Can you work these out from the model? Positions are in its coordinate system, mm. Face numbers are marked on the shaded views. A direction names the side the tool comes from. Give positions to 0.01 mm unless a question says otherwise; leave off trailing zeros. Order: outer loops, then holes, each group sorted by start corner. A loop starts at its lowest first (then second) coordinate and runs counter-clockwise, first axis right, second up. Notation, with made-up numbers: (-12, -1.5) - (-4, -1.5) arc R17 cw to (-4, 31.5) - close; hole circle Ø7 at (-26.5, -29). An arc over 180 degrees is marked (long way). Return JSON: item names as keys, results as strings.
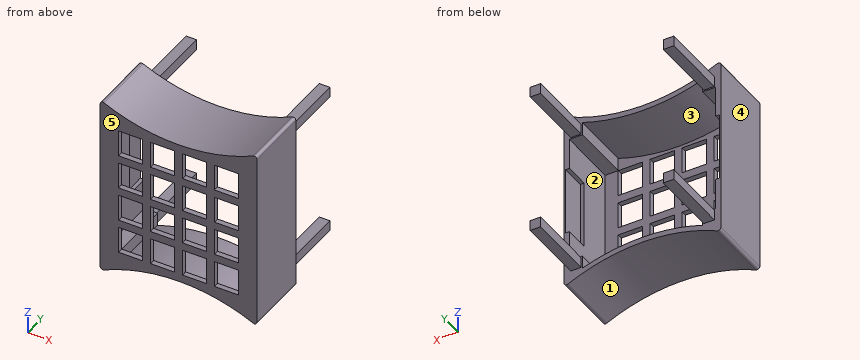
```python
from build123d import *

# Parameters (mm, degrees)
RESSALTO_EXTRUS_O1_DEPTH = 25
CASCA1_T                 = -2
ESBO_O3_W                = 4
ESBO_O3_H                = 4
RESSALTO_EXTRUS_O2_DEPTH = 23
ESBO_O3_3_W              = 4
ESBO_O3_3_H              = 4
RESSALTO_EXTRUS_O3_DEPTH = 49
FILETE1_R                = 1
CORTE_EXTRUS_O1_START    = -0.5
ESBO_O4_W                = 26
ESBO_O4_H                = 9.5
ESBO_O4_H_2              = 3.5
CORTE_EXTRUS_O1_DEPTH    = 59
ESBO_O5_W                = 9.25
ESBO_O5_H                = 10.19955009
CORTE_EXTRUS_O2_DEPTH    = 10


with BuildPart() as part:
    # Esboço2 → Ressalto-extrusão1 (new body)
    with BuildSketch(Plane(origin=(0, 0, 0), x_dir=(1, 0, 0), z_dir=(0, 1, 0))):
        with BuildLine():
            Line((-30, 35), (-30, -35))
            ThreePointArc((-30, -35), (0, -28), (30, -35))
            Line((30, -35), (30, 35))
            ThreePointArc((30, 35), (0, 28), (-30, 35))
        make_face()
    extrude(amount=RESSALTO_EXTRUS_O1_DEPTH)

    # Casca1
    casca1_openings = [part.faces().sort_by_distance(p)[0] for p in [
        (0, 25, 0),
    ]]
    offset(amount=CASCA1_T, openings=casca1_openings, kind=Kind.INTERSECTION)

    # Esboço3 → Ressalto-extrusão2 (add)
    # profile 1 of 4: a face of its own
    with BuildSketch(Plane(origin=(0, 2, 0), x_dir=(1, 0, 0), z_dir=(0, 1, 0))):
        with BuildLine():
            Line((23, 24.89910018), (28, 24.89910018))
            Line((28, 24.89910018), (28, 31.863527853))
            ThreePointArc((28, 31.863527853), (25.518909538, 30.833184124), (23, 29.89910018))
            Line((23, 29.89910018), (23, 24.89910018))
        make_face()
        with Locations((25.5, 27.39910018)):
            Rectangle(ESBO_O3_W, ESBO_O3_H, mode=Mode.SUBTRACT)
    # profile 2 of 4: a face of its own
    with BuildSketch(Plane(origin=(0, 2, 0), x_dir=(1, 0, 0), z_dir=(0, 1, 0))):
        with BuildLine():
            Line((28, -31.863527853), (28, -24.89910018))
            Line((28, -24.89910018), (23, -24.89910018))
            Line((23, -24.89910018), (23, -29.89910018))
            ThreePointArc((23, -29.89910018), (25.518909538, -30.833184124), (28, -31.863527853))
        make_face()
        with Locations((25.5, -27.39910018)):
            Rectangle(ESBO_O3_W, ESBO_O3_H, mode=Mode.SUBTRACT)
    # profile 3 of 4: a face of its own
    with BuildSketch(Plane(origin=(0, 2, 0), x_dir=(1, 0, 0), z_dir=(0, 1, 0))):
        with BuildLine():
            Line((-23, 24.89910018), (-23, 29.89910018))
            ThreePointArc((-23, 29.89910018), (-25.518909538, 30.833184124), (-28, 31.863527853))
            Line((-28, 31.863527853), (-28, 24.89910018))
            Line((-28, 24.89910018), (-23, 24.89910018))
        make_face()
        with Locations((-25.5, 27.39910018)):
            Rectangle(ESBO_O3_W, ESBO_O3_H, mode=Mode.SUBTRACT)
    # profile 4 of 4: a face of its own
    with BuildSketch(Plane(origin=(0, 2, 0), x_dir=(1, 0, 0), z_dir=(0, 1, 0))):
        with BuildLine():
            ThreePointArc((-28, -31.863527853), (-25.518909538, -30.833184124), (-23, -29.89910018))
            Line((-23, -29.89910018), (-23, -24.89910018))
            Line((-23, -24.89910018), (-28, -24.89910018))
            Line((-28, -24.89910018), (-28, -31.863527853))
        make_face()
        with Locations((-25.5, -27.39910018)):
            Rectangle(ESBO_O3_W, ESBO_O3_H, mode=Mode.SUBTRACT)
    extrude(amount=RESSALTO_EXTRUS_O2_DEPTH)

    # Esboço3<3> → Ressalto-extrusão3 (add)
    with BuildSketch(Plane(origin=(0, 2, 0), x_dir=(1, 0, 0), z_dir=(0, 1, 0))):
        with Locations((25.5, 27.39910018)):
            Rectangle(ESBO_O3_3_W, ESBO_O3_3_H)
        with Locations((25.5, -27.39910018)):
            Rectangle(ESBO_O3_3_W, ESBO_O3_3_H)
        with Locations((-25.5, 27.39910018)):
            Rectangle(ESBO_O3_3_W, ESBO_O3_3_H)
        with Locations((-25.5, -27.39910018)):
            Rectangle(ESBO_O3_3_W, ESBO_O3_3_H)
    extrude(amount=RESSALTO_EXTRUS_O3_DEPTH)

    # Filete1
    filete1_edges = [part.edges().sort_by_distance(p)[0] for p in [
        (-30, 12.5, 35),
        (-30, 12.5, -35),
        (30, 12.5, -35),
        (30, 12.5, 35),
    ]]
    fillet(filete1_edges, radius=FILETE1_R)

    # Esboço4 → Corte-extrusão1 (cut)
    with BuildSketch(Plane(origin=(30, 0, 0), x_dir=(0, 0, -1), z_dir=(1, 0, 0)).offset(CORTE_EXTRUS_O1_START)):
        with Locations((0, 20.25)):
            Rectangle(ESBO_O4_W, ESBO_O4_H)
        with Locations((0, 26.75)):
            Rectangle(ESBO_O4_W, ESBO_O4_H_2)
    extrude(amount=-CORTE_EXTRUS_O1_DEPTH, mode=Mode.SUBTRACT)

    # Esboço5 → Corte-extrusão2 (cut)
    with BuildSketch(Plane(origin=(0, 2, 0), x_dir=(1, 0, 0), z_dir=(0, 1, 0))):
        with Locations((-18.375, 19.799325135)):
            Rectangle(ESBO_O5_W, ESBO_O5_H)
        Polygon((-13.75, 4.5), (-13.75, 11.69955009), (-23, 11.69955009), (-23, 4.5), (-23, 1.5), (-13.75, 1.5), align=None)
        with Locations((-6.125, 6.599775045)):
            Rectangle(ESBO_O5_W, ESBO_O5_H)
        Polygon((-10.75, 24.89910018), (-10.75, 14.69955009), (-4.5, 14.69955009), (-1.5, 14.69955009), (-1.5, 24.89910018), (-4.5, 24.89910018), align=None)
        Polygon((-23, -11.69955009), (-13.75, -11.69955009), (-13.75, -4.5), (-13.75, -1.5), (-23, -1.5), (-23, -4.5), align=None)
        with Locations((-6.125, -6.599775045)):
            Rectangle(ESBO_O5_W, ESBO_O5_H)
        with Locations((-18.375, -19.799325135)):
            Rectangle(ESBO_O5_W, ESBO_O5_H)
        Polygon((-1.5, -14.69955009), (-4.5, -14.69955009), (-10.75, -14.69955009), (-10.75, -24.89910018), (-4.5, -24.89910018), (-1.5, -24.89910018), align=None)
        Polygon((10.75, -14.69955009), (1.5, -14.69955009), (1.5, -24.89910018), (4.5, -24.89910018), (10.75, -24.89910018), align=None)
        with Locations((18.375, -19.799325135)):
            Rectangle(ESBO_O5_W, ESBO_O5_H)
        Polygon((13.75, -1.5), (13.75, -11.69955009), (23, -11.69955009), (23, -4.5), (23, -1.5), align=None)
        with Locations((6.125, -6.599775045)):
            Rectangle(ESBO_O5_W, ESBO_O5_H)
        with Locations((6.125, 6.599775045)):
            Rectangle(ESBO_O5_W, ESBO_O5_H)
        Polygon((13.75, 11.69955009), (13.75, 1.5), (23, 1.5), (23, 4.5), (23, 11.69955009), align=None)
        with Locations((18.375, 19.799325135)):
            Rectangle(ESBO_O5_W, ESBO_O5_H)
        Polygon((4.5, 14.69955009), (10.75, 14.69955009), (10.75, 24.89910018), (4.5, 24.89910018), (1.5, 24.89910018), (1.5, 14.69955009), align=None)
    extrude(amount=-CORTE_EXTRUS_O2_DEPTH, mode=Mode.SUBTRACT)


solid = part.part
```
1. Suppose I cut it at B-B (y = 8). List the corners of the cut face in (x, z) for me, plus the area to 3 significant figures.
Checks:
{"outline": "(-30, -33.41) arc R1 ccw to (-28.58, -34.32) arc R67.79 cw to (28.58, -34.32) arc R1 ccw to (30, -33.41) - (30, 33.41) arc R1 ccw to (28.58, 34.32) arc R67.79 cw to (-28.58, 34.32) arc R1 ccw to (-30, 33.41) - close; hole (-28, -24.9) - (-23, -24.9) - (-23, -29.9) arc R69.79 cw to (23, -29.9) - (23, -24.9) - (28, -24.9) - (28, 24.9) - (23, 24.9) - (23, 29.9) arc R69.79 cw to (-23, 29.9) - (-23, 24.9) - (-28, 24.9) - close", "area": "623 mm^2"}
2. On a 3-axis mill with a long thin cutter (end or side, diameter ignored), from which of +Z, -Z, +X, -X, +Y, -Y can I reach the whole of each face in a straight line? I mean the marked faces 1 and 2. Say none if no direction works.
Checks:
{"face 1": "-Z, +Y, -Y", "face 2": "+Y"}
3. Suppose I cut it at C-C (y = 46). List the corners of the cut face in (x, z) for me, plus the area to 3 significant figures.
Checks:
{"outline": "(-27.5, -29.4) - (-23.5, -29.4) - (-23.5, -25.4) - (-27.5, -25.4) - close; (-27.5, 25.4) - (-23.5, 25.4) - (-23.5, 29.4) - (-27.5, 29.4) - close; (23.5, -29.4) - (27.5, -29.4) - (27.5, -25.4) - (23.5, -25.4) - close; (23.5, 25.4) - (27.5, 25.4) - (27.5, 29.4) - (23.5, 29.4) - close", "area": "64.0 mm^2"}
4. For pin 1 Ø4 at (x, z) = (-23.5, 15) entering from +Y; pin 2 Ø2 at (x, z) = (-2.5, 26.5) entering from +Y; pin 3 Ø3 at (x, y) = (4.5, 17.5) entering from +Z, each with a flat end and sliding along its axis, tell me the tip position at first contact or that it passes through.
Checks:
{"pin 1": "y = 2", "pin 2": "y = 25", "pin 3": "z = 28.27"}
5. Suppose I cut it at D-D (x = 7). List the corners of the cut face in (y, z) for me, plus the area to 3 significant figures.
Checks:
{"outline": "(0, -28.36) - (25, -28.36) - (25, -26.35) - (2, -26.35) - (2, -24.9) - (0, -24.9) - close; (0, -14.7) - (2, -14.7) - (2, -11.7) - (0, -11.7) - close; (0, -1.5) - (2, -1.5) - (2, 1.5) - (0, 1.5) - close; (0, 11.7) - (2, 11.7) - (2, 14.7) - (0, 14.7) - close; (0, 24.9) - (2, 24.9) - (2, 26.35) - (25, 26.35) - (25, 28.36) - (0, 28.36) - close", "area": "124 mm^2"}
6. Thinking about a two-plate mould opening in X: for the marked faces 3, 4 and 5, which applies, +X half, -X half, draft (parallel to the pull), parting line (faces both ways), or undercut?
Checks:
{"face 3": "undercut", "face 4": "-X half", "face 5": "draft"}
7. Suppose I cut it at A-A (z = -3). List the corners of the cut face in (x, y) for me.
Checks:
{"outline": "(-30, 0) - (-23, 0) - (-23, 2) - (-28, 2) - (-28, 15.5) - (-29.5, 15.5) - (-29.5, 25) - (-30, 25) - close; (-13.75, 0) - (-10.75, 0) - (-10.75, 2) - (-13.75, 2) - close; (-1.5, 0) - (1.5, 0) - (1.5, 2) - (-1.5, 2) - close; (10.75, 0) - (13.75, 0) - (13.75, 2) - (10.75, 2) - close; (23, 0) - (30, 0) - (30, 25) - (29.5, 25) - (29.5, 15.5) - (28, 15.5) - (28, 2) - (23, 2) - close"}
8. If I drill on L1, parallel to X at y = 46.5, z = 27; L2, parallel to X at y = 18.5, z = -19.5; L3, parallel to Z at x = -27, y = 44, over which ranges is the centre line in solid material (lowest first)? Write a range as [from, to].
Checks:
{"L1": "[-27.5, -23.5], [23.5, 27.5]", "L2": "[-30, -28], [28, 30]", "L3": "[-29.4, -25.4], [25.4, 29.4]"}
